```python
from build123d import *

# Parameters (mm, degrees)
BOSS_EXTRUDE1_DEPTH = 4
SKETCH3_R           = 3.41
CUT_EXTRUDE1_DEPTH  = 137.073509545
SKETCH4_R           = 6.5
CUT_EXTRUDE2_DEPTH  = 137.073509545


with BuildPart() as part:
    # Sketch2 → Boss-Extrude1 (new body)
    with BuildSketch(Plane(origin=(0, 0, 0), x_dir=(1, 0, 0), z_dir=(0, 1, 0))):
        Polygon((-110, 76), (-110, 25), (-106, 25), (-106, -25), (-110, -25), (-110, -76), (-75, -76), (-75, -80), (-25, -80), (-25, -76), (25, -76), (25, -80), (75, -80), (75, -76), (110, -76), (110, -25), (106, -25), (106, 25), (110, 25), (110, 76), (75, 76), (75, 80), (25, 80), (25, 76), (-25, 76), (-25, 80), (-75, 80), (-75, 76), align=None)
    extrude(amount=BOSS_EXTRUDE1_DEPTH)

    # Sketch3 → Cut-Extrude1 (cut, through all)
    with BuildSketch(Plane(origin=(0, 4, 0), x_dir=(1, 0, 0), z_dir=(0, 1, 0))):
        with Locations(Location((90, -60, 0), (0, 0, 270))):
            Circle(SKETCH3_R)
        with Locations(Location((-3, -60, 0), (0, 0, 270))):
            Circle(SKETCH3_R)
        with Locations(Location((-3, 40, 0), (0, 0, 270))):
            Circle(SKETCH3_R)
    extrude(amount=-CUT_EXTRUDE1_DEPTH, mode=Mode.SUBTRACT)

    # Sketch4 → Cut-Extrude2 (cut, through all)
    with BuildSketch(Plane(origin=(0, 4, 0), x_dir=(1, 0, 0), z_dir=(0, 1, 0))):
        with Locations(Location((33.5, 59, 0), (0, 0, 270))):
            Circle(SKETCH4_R)
    extrude(amount=-CUT_EXTRUDE2_DEPTH, mode=Mode.SUBTRACT)


solid = part.part
```
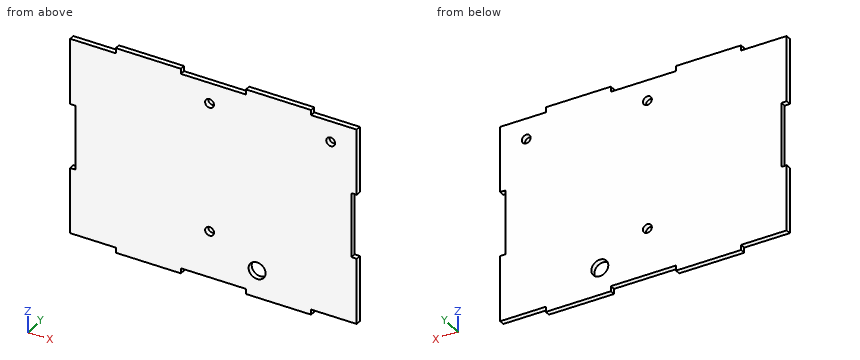
Design review of the part built by this model. Coordinates are the model's own, in mm. Coordinates: 2 decimals unless noted, no trailing zeros. Write each loop counter-clockwise with the first axis right and the second up, starting at its lowest first coordinate (ties: lowest second). Pieces come first, ordered by that corner, then holes.
1) Add section C-C (z = 60). Write out the cut boundary in (x, y).
2) Add section B-B (x = 90). Write out the cut boundary in (y, z), plus the area to 3 significant figures.
3) Add section A-A (z = -59). Write out the cut boundary in (x, y).
4) To check wall thickness, follow L1, parallel to X at y = 1.35, z = -40; L2, parallel to X at y = 1.4, z = 60; L3, parallel to X at y = 2.1, z = 15.5. State the ranges of each line that lie inside material, in increasing order.
5) Add section D-D (y = 0.8). State how many separate pieces and enclosed holes the cut face has, plus the area to 3 significant figures.
6) Insertion check: pin 1 (11 mm diameter, centred on x = -3, z = 60, fed in from -Y); pin 2 (2 mm diameter, centred on y = 1.5, z = -77.5, fed in from -X); pin 3 (1.2 mm diameter, centred on y = 1, z = 79, fed in from +X); pin 4 (2 mm diameter, centred on y = 2, z = -5, fed in from +X). Each pin has a flat end and moves straight along its axis. Give the tip position at first contact, or say it passes through.
Check result:
1. outline: (-110, 0) - (-6.41, 0) - (-6.41, 4) - (-110, 4) - close; (0.41, 0) - (86.59, 0) - (86.59, 4) - (0.41, 4) - close; (93.41, 0) - (110, 0) - (110, 4) - (93.41, 4) - close
2. outline: (0, -76) - (4, -76) - (4, 56.59) - (0, 56.59) - close; (0, 63.41) - (4, 63.41) - (4, 76) - (0, 76) - close
2. area: 581 mm2
3. outline: (-110, 0) - (27, 0) - (27, 4) - (-110, 4) - close; (40, 0) - (110, 0) - (110, 4) - (40, 4) - close
4. L1: x = -110 to -6.41, 0.41 to 110
4. L2: x = -110 to -6.41, 0.41 to 86.59, 93.41 to 110
4. L3: x = -106 to 106
5. separate pieces: 1
5. enclosed holes: 4
5. area: 33,600 mm2
6. pin 1: stops at y = 0
6. pin 2: stops at x = -75
6. pin 3: stops at x = 75
6. pin 4: stops at x = 106
